```python
from build123d import *

# Parameters (mm, degrees)
EXTRUDE_1_DEPTH     = 5
CUT_EXTRUDE_1_DEPTH = 5
SKETCH_4_W          = 5
SKETCH_4_H          = 20
EXTRUDE_2_DEPTH     = 5


with BuildPart() as part:
    # 草图1 → 凸台-拉伸1 (new body)
    with BuildSketch(Plane.XY):
        Polygon((175, 10), (0, 10), (-175, 10), (-175, -10), (175, -10), align=None)
    extrude(amount=EXTRUDE_1_DEPTH)

    # 草图3 → 切除-拉伸1 (cut)
    with BuildSketch(Plane(origin=(0, 0, 0), x_dir=(-1, 0, 0), z_dir=(0, 0, -1))):
        with BuildLine():
            Line((-165, 5), (-165, 0))
            Line((-165, 0), (-162.25, 0))
            Line((-162.25, 0), (-162.25, 5))
            ThreePointArc((-162.25, 5), (-163.055456352, 6.944543648), (-165, 7.75))
            Line((-165, 7.75), (-165, 5))
        make_face()
        with BuildLine():
            Line((-167.75, 5), (-167.75, 0))
            Line((-167.75, 0), (-165, 0))
            Line((-165, 0), (-165, 5))
            Line((-165, 5), (-165, 7.75))
            ThreePointArc((-165, 7.75), (-166.944543648, 6.944543648), (-167.75, 5))
        make_face()
        with BuildLine():
            Line((-165, 0), (-167.75, 0))
            Line((-167.75, 0), (-167.75, -5))
            ThreePointArc((-167.75, -5), (-166.944543648, -6.944543648), (-165, -7.75))
            Line((-165, -7.75), (-165, -5))
            Line((-165, -5), (-165, 0))
        make_face()
        with BuildLine():
            Line((-162.25, 0), (-165, 0))
            Line((-165, 0), (-165, -5))
            Line((-165, -5), (-165, -7.75))
            ThreePointArc((-165, -7.75), (-163.055456352, -6.944543648), (-162.25, -5))
            Line((-162.25, -5), (-162.25, 0))
        make_face()
        with BuildLine():
            Line((-155, 0), (-157.75, 0))
            ThreePointArc((-157.75, 0), (-156.944543648, -1.944543648), (-155, -2.75))
            Line((-155, -2.75), (155, -2.75))
            ThreePointArc((155, -2.75), (156.944543648, -1.944543648), (157.75, 0))
            Line((157.75, 0), (155, 0))
            Line((155, 0), (-155, 0))
        make_face()
        with BuildLine():
            ThreePointArc((-155, 2.75), (-156.944543648, 1.944543648), (-157.75, 0))
            Line((-157.75, 0), (-155, 0))
            Line((-155, 0), (155, 0))
            Line((155, 0), (157.75, 0))
            ThreePointArc((157.75, 0), (156.944543648, 1.944543648), (155, 2.75))
            Line((155, 2.75), (-155, 2.75))
        make_face()
        with BuildLine():
            Line((165, 5), (165, 0))
            Line((165, 0), (167.75, 0))
            Line((167.75, 0), (167.75, 5))
            ThreePointArc((167.75, 5), (166.944543648, 6.944543648), (165, 7.75))
            Line((165, 7.75), (165, 5))
        make_face()
        with BuildLine():
            Line((162.25, 5), (162.25, 0))
            Line((162.25, 0), (165, 0))
            Line((165, 0), (165, 5))
            Line((165, 5), (165, 7.75))
            ThreePointArc((165, 7.75), (163.055456352, 6.944543648), (162.25, 5))
        make_face()
        with BuildLine():
            Line((165, 0), (162.25, 0))
            Line((162.25, 0), (162.25, -5))
            ThreePointArc((162.25, -5), (163.055456352, -6.944543648), (165, -7.75))
            Line((165, -7.75), (165, -5))
            Line((165, -5), (165, 0))
        make_face()
        with BuildLine():
            Line((167.75, 0), (165, 0))
            Line((165, 0), (165, -5))
            Line((165, -5), (165, -7.75))
            ThreePointArc((165, -7.75), (166.944543648, -6.944543648), (167.75, -5))
            Line((167.75, -5), (167.75, 0))
        make_face()
    extrude(amount=-CUT_EXTRUDE_1_DEPTH, mode=Mode.SUBTRACT)

    # 草图4 → 凸台-拉伸2 (add)
    with BuildSketch(Plane(origin=(0, 0, 0), x_dir=(-1, 0, 0), z_dir=(0, 0, -1))):
        with Locations((-177.5, 0)):
            Rectangle(SKETCH_4_W, SKETCH_4_H)
        with Locations((177.5, 0)):
            Rectangle(SKETCH_4_W, SKETCH_4_H)
    extrude(amount=-EXTRUDE_2_DEPTH)


solid = part.part
```
Geometry check sheet. Reference: the model listing, model coordinates, mm. Coordinates: 2 decimals unless noted, no trailing zeros. Order: outer loops, then holes, each group sorted by start corner. A loop starts at its lowest first (then second) coordinate and runs counter-clockwise, first axis right, second up. Notation, with made-up numbers: (47, 80.5) - (88, 80.5) arc R22 ccw to (88, 110.5) - close; hole circle Ø1 at (18, 68.5). An arc over 180 degrees is marked (long way). Answer as a JSON object with one key per item and string values. Group by question number.
Item 1: Sectioned sample at A-A, the plane x = -77. Record the cut outline in (y, z), and give its area (3 significant figures).
Item 2: Scan lines: probe 1 along X at (y, z) = (-3, 0.25); probe 2 along X at (y, z) = (5.25, 1.65); probe 3 along Y at (x, z) = (56, 3.35). Record each from-to range of solid material in increasing order.
Item 3: Sectioned sample at B-B, the plane z = 3.65. Record the cut outline in (x, y), and give its area (3 significant figures).
Resolved:
{
 "1": {"outline": "(-10, 0) - (-2.75, 0) - (-2.75, 5) - (-10, 5) - close; (2.75, 0) - (10, 0) - (10, 5) - (2.75, 5) - close", "area": "72.5 mm^2"},
 "2": {"probe 1": "-180 to -167.75, -162.25 to 162.25, 167.75 to 180", "probe 2": "-180 to -167.74, -162.26 to 162.26, 167.74 to 180", "probe 3": "-10 to -2.75, 2.75 to 10"},
 "3": {"outline": "(-180, -10) - (180, -10) - (180, 10) - (-180, 10) - close; hole (-167.75, -5) arc R2.75 ccw to (-162.25, -5) - (-162.25, 5) arc R2.75 ccw to (-167.75, 5) - close; hole (-155, -2.75) - (155, -2.75) arc R2.75 ccw to (155, 2.75) - (-155, 2.75) arc R2.75 ccw to start; hole (162.25, -5) arc R2.75 ccw to (167.75, -5) - (167.75, 5) arc R2.75 ccw to (162.25, 5) - close", "area": "5,310 mm^2"}
}
